```python
from build123d import *

# Parameters (mm, degrees)
F3_DEPTH = 0.2
F4_COUNT = 4


# Not quite as in the source:
# - a feature names something its author has since deleted; it is built from what else it names


with BuildPart() as f1:
    # F0 (on Front) → F1 (revolve)
    with BuildSketch(Plane.XZ):
        with BuildLine():
            Line((0, 22.2222222222), (0, 0))
            Line((0, 0), (1.1284722222, 0))
            Line((1.1284722222, 0), (1.2847222222, 3.2638888889))
            Line((1.2847222222, 3.2638888889), (1.2847222222, 18.5416666667))
            ThreePointArc((1.2847222222, 18.5416666667), (1.074687159, 20.2927272078), (0.4564979348, 21.9444444444))
            ThreePointArc((0.4564979348, 21.9444444444), (0.2671847948, 22.1473201826), (0, 22.2222222222))
        make_face()
    revolve(axis=Axis((0, 0, 11.1111111111), (0, 0, 1)))

    # F2 (on Front) → F3 (join, symmetric)
    with BuildSketch(Plane.XZ):
        Polygon((0, 3.2638888889), (0, 0), (3.0208333333, 0), (2.8125, 2.5694444444), (0.4, 2.5694444444), (0.4, 3.2638888889), align=None)
        with BuildLine():
            Line((0, 16.0250628992), (0, 3.2638888889))
            Line((0, 3.2638888889), (0.4, 3.2638888889))
            Line((0.4, 3.2638888889), (0.4, 3.6805555556))
            Line((0.4, 3.6805555556), (2.7224099099, 3.6805555556))
            Line((2.7224099099, 3.6805555556), (1.7708333333, 15.4166666667))
            ThreePointArc((1.7708333333, 15.4166666667), (1.5598257716, 15.8497451466), (1.1111111111, 16.0250628992))
            Line((1.1111111111, 16.0250628992), (0, 16.0250628992))
        make_face()
    extrude(amount=F3_DEPTH, both=True)

    # F4: F1 ×4 about axis
    f4_axis = Axis((0, 0, 3.2638888889), (0, 0, 1))


with BuildPart() as f1_1:
    add(f1.part)
    for i in range(1, F4_COUNT):
        add(f1.part.rotate(f4_axis, i * 360 / F4_COUNT))


solid = f1_1.part
```
Here's how the part is built. I have some questions about the finished solid (model axes, mm). A direction names the side the tool comes from. Round coordinates to 2 decimals unless told otherwise and drop trailing zeros. Write each loop counter-clockwise with the first axis right and the second up, starting at its lowest first coordinate (ties: lowest second). Pieces come first, ordered by that corner, then holes. Notation, with made-up numbers: M 23,18 L 81,18 A32 cw 81,50 Z; hole C 20.25,17.5 d8. An arc over 180 degrees is marked long. Answer as CSV lines item,"result". Start each with the question number.
1. I need wall thicknesses on probe 1 along Y at (x, z) = (2, 3.75); probe 2 along Y at (x, z) = (0, 16.75). Which ranges of each line are inside material? Lowest first, please.
2. Suppose I cut it at D-D on z = 12.25. Write out the boundary of the cut face in (x, y).
3. Suppose I cut it at B-B on y = -2. Write out the boundary of the cut face in (x, z).
4. I'm going to push flat-ended pins straight in: pin 1 Ø1 at (x, z) = (-1.5, 1.5) entering from -Y; pin 2 Ø0.6 at (x, z) = (1.5, 0.5) entering from +Y; pin 3 Ø2 at (x, y) = (2, 2) entering from +Z; pin 4 Ø0.6 at (y, z) = (2.5, 1) entering from -X. Where does each tip first touch, or does it pass through?
5. Suppose I cut it at A-A on x = 2.25. Write out the boundary of the cut face in (y, z), then the cut area to 3 significant figures.
6. On a 3-axis mill with a long thin cutter (end or side, diameter ignored), from which of +Z, -Z, +X, -X, +Y, -Y can I reach the whole of each face in a straight line? I mean faces 1 (the flat face through (2, -0.2, 9)), 2 (the flat face through (-0.2, -2, 9)), 3 (the flat face through (-0.003, -2.253, 9.466)), 4 (the flat face through (2, 0.2, 9)), 5 (the flat face through (-0.2, 2, 9)). Say none if no direction works.
7. Suppose I cut it at C-C on z = 9.75. Write out the boundary of the cut face in (x, y).
Check result:
1,probe 1,"y = -0.2 to 0.2"
1,probe 2,"y = -1.28 to 1.28"
2,outline,"M -2.03,-0.2 L -1.27,-0.2 A1.28 ccw -0.2,-1.27 L -0.2,-2.03 L 0.2,-2.03 L 0.2,-1.27 A1.28 ccw 1.27,-0.2 L 2.03,-0.2 L 2.03,0.2 L 1.27,0.2 A1.28 ccw 0.2,1.27 L 0.2,2.03 L -0.2,2.03 L -0.2,1.27 A1.28 ccw -1.27,0.2 L -2.03,0.2 Z"
3,outline,"M -0.2,0 L 0.2,0 L 0.2,2.57 L -0.2,2.57 Z; M -0.2,3.68 L 0.2,3.68 L 0.2,12.59 L -0.2,12.59 Z"
4,pin 1,"stops at y = -0.67"
4,pin 2,"stops at y = 0.2"
4,pin 3,"passes through"
4,pin 4,"stops at x = -0.2"
5,outline,"M -0.2,0 L 0.2,0 L 0.2,2.57 L -0.2,2.57 Z; M -0.2,3.68 L 0.2,3.68 L 0.2,9.51 L -0.2,9.51 Z"
5,area,"3.36 mm2"
6,face 1,"+Z, -Z, +X, -Y"
6,face 2,"+Z, -Z, -X, -Y"
6,face 3,"+Z, +X, -X, -Y"
6,face 4,"+Z, -Z, +X, +Y"
6,face 5,"+Z, -Z, -X, +Y"
7,outline,"M -2.23,-0.2 L -1.27,-0.2 A1.28 ccw -0.2,-1.27 L -0.2,-2.23 L 0.2,-2.23 L 0.2,-1.27 A1.28 ccw 1.27,-0.2 L 2.23,-0.2 L 2.23,0.2 L 1.27,0.2 A1.28 ccw 0.2,1.27 L 0.2,2.23 L -0.2,2.23 L -0.2,1.27 A1.28 ccw -1.27,0.2 L -2.23,0.2 Z"
